Autodesk Inventor part; units mm, degrees
ref_plane "YZ Plane" through (0, 0, 0) normal (1, 0, 0) x (0, 1, 0)
ref_plane "XZ Plane" through (0, 0, 0) normal (0, 1, 0) x (-1, 0, 0)
ref_plane "XY Plane" through (0, 0, 0) normal (0, 0, 1) x (1, 0, 0)
sketch "Sketch2" plane through (0, 0, 0) normal (1, 0, 0) x (0, 1, 0)
  line L0 (0, 0) -> (920, 0)
  line L1 (920, 0) -> (920, -50)
  line L2 (920, -50) -> (0, -50)
  line L3 (0, -50) -> (0, 0)
  line L4 (920, -50) -> (883.2713, 0) construction
  line L5 (920, 0) -> (851.9332, -50)
  line L6 (0, 0) -> (36.7287, -50)
  dimension "d28" = 920
  dimension "d29" = 50
  dimension "d31" = 36.3
  dimension "d32" = 53.7
  dimension "d36" = 53.7
extrude "Plate2" add sketch "Sketch2" along normal blind 3 contours L0 L5 L2 L6
chamfer "Corner Chamfer1" distance 3 angle 45 2 edges at (1.5, 920, 0) (1.5, 0, 0)
fillet "Corner Round1" radius 6 2 edges at (1.5, 36.7287, -50) (1.5, 851.9332, -50)
sketch "Sketch3" plane through (3, 0, 0) normal (1, 0, 0) x (0, 0, -1)
  line L0 (24, 217.54) -> (50, 217.54)
  line L1 (50, 217.54) -> (50, 220.54)
  line L2 (50, 220.54) -> (24, 220.54)
  line L3 (24, 220.54) -> (24, 217.54)
  line L4 (50, 849.9663) -> (50, 39.766)
  line L5 (50, 219.04) -> (0, 219.04) construction
  line L6 (0, 3) -> (0, 917)
  line L7 (50, 599.04) -> (0, 599.04) construction
  line L8 (24, 597.54) -> (50, 597.54)
  line L9 (50, 597.54) -> (50, 600.54)
  line L10 (50, 600.54) -> (24, 600.54)
  line L11 (24, 600.54) -> (24, 597.54)
  point P0 (0, 0)
  dimension "d39" = 26
  dimension "d40" = 3
  dimension "d41" = 219.04
  dimension "d42" = 599.04
  dimension "d43" = 3
  dimension "d44" = 26
extrude "Extrusion1" cut sketch "Sketch3" against normal through all
sketch "Sketch4" plane through (3, 0, 0) normal (1, 0, 0) x (0, 0, -1)
  line L0 (17.0121, 486.3959) -> (33.8114, 486.3959) construction
  line L1 (33.8114, 486.3959) -> (33.8114, 335.9678) construction
  line L2 (33.8114, 335.9678) -> (17.0121, 335.9678) construction
  line L3 (17.0121, 335.9678) -> (17.0121, 486.3959) construction
  point P0 (0, 0)
mark "Mark1"
equation "\"d36\" = d32"
equation "\"d40\" = Thickness"
equation "\"d43\" = Thickness"
equation "\"d44\" = d39"
equation "\"d30\" = Thickness"
equation "\"BendReliefWidth\" = Thickness"
equation "\"BendReliefDepth\" = 0.5 * Thickness"
equation "\"CornerReliefSize\" = 4 * Thickness"
equation "\"MinimumRemnant\" = 2 * Thickness"
equation "\"TransitionRadius\" = BendRadius"
equation "\"JacobiRadiusSize\" = BendRadius"
equation "\"GapSize\" = Thickness"
properties part number "MSC 110 STRINGER CONE" material "Stainless Steel"
The listing builds one solid part. Answer for the finished solid, in the listing's coordinates (mm). Round coordinates to 2 decimals unless told otherwise and drop trailing zeros. Loops run counter-clockwise (first coordinate to the right, second up) from the corner with the lowest first, then second, coordinate; pieces in that order, holes last.
1) Consider line 1 (Y direction, x = 2.65, z = -39); line 2 (Y direction, x = 2.3, z = -36); line 3 (Y direction, x = 0.95, z = -5). Determine where each line is inside the solid, lowest interval first.
Outcome:
line 1: y = 28.65 to 217.54, 220.54 to 597.54, 600.54 to 866.91
line 2: y = 26.44 to 217.54, 220.54 to 597.54, 600.54 to 870.99
line 3: y = 3.67 to 913.19
2) A cutting plane is placed at A-A on x = 2.3. Determine the outline of the cut face in (y, z), plus the area to 3 significant figures.
Outcome:
outline: (1.78, -2.42) - (34.93, -47.55) arc R6 ccw to (39.77, -50) - (217.54, -50) - (217.54, -24) - (220.54, -24) - (220.54, -50) - (597.54, -50) - (597.54, -24) - (600.54, -24) - (600.54, -50) - (849.97, -50) arc R6 ccw to (853.52, -48.84) - (917.58, -1.78) - (917, 0) - (3, 0) - close
area: 43,200 mm2
3) Given P1, Ø1.5, axis at x = 2, z = -39, coming from the +Y side; P2, Ø1.5, axis at x = 2.5, z = -10, coming from the +Y side; P3, Ø1, axis at x = 0.5, z = -24.5, coming from the +Y side; P4, Ø10, axis at y = 199.5, z = -25.5, coming from the -X side, each flat-ended and moving along its own axis, determine where each tip first touches the part or whether it passes through.
Outcome:
P1: stops at y = 867.93
P2: stops at y = 907.41
P3: stops at y = 887.33
P4: stops at x = 0
4) A cutting plane is placed at B-B on z = -38.5. Determine the outline of the cut face in (x, y).
Outcome:
outline: (0, 28.28) - (3, 28.28) - (3, 217.54) - (0, 217.54) - close; (0, 220.54) - (3, 220.54) - (3, 597.54) - (0, 597.54) - close; (0, 600.54) - (3, 600.54) - (3, 867.59) - (0, 867.59) - close
